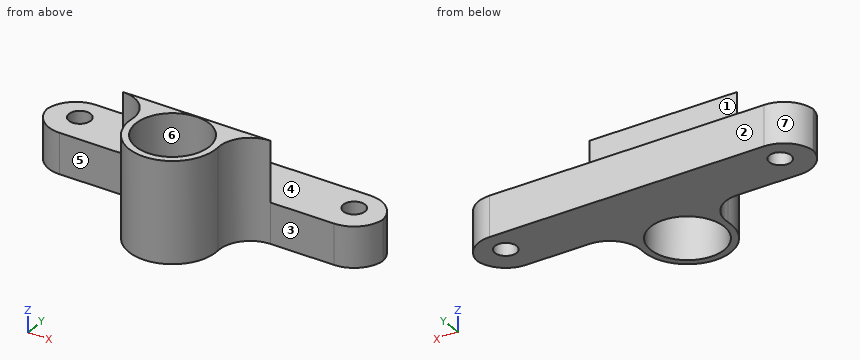
from build123d import *

# Parameters (mm, degrees)
F0_R     = 1.75
F0_R_2   = 5.9
F1_DEPTH = 6.5
F2_DEPTH = 16.2


with BuildPart() as f1:
    # F0 (on Top) → F1 (new body)
    with BuildSketch(Plane.XY):
        with BuildLine():
            Line((7.780111, 20.456612), (-36.719889, 20.456612))
            ThreePointArc((-36.719889, 20.456612), (-40.073991, 19.164712), (-41.694827, 15.956612))
            ThreePointArc((-41.694827, 15.956612), (-40.073991, 12.748513), (-36.719889, 11.456612))
            Line((-36.719889, 11.456612), (-26.42815, 11.456612))
            Line((-26.42815, 11.456612), (-2.511629, 11.456612))
            Line((-2.511629, 11.456612), (7.780111, 11.456612))
            ThreePointArc((7.780111, 11.456612), (11.134213, 12.748513), (12.755048, 15.956612))
            ThreePointArc((12.755048, 15.956612), (11.134213, 19.164712), (7.780111, 20.456612))
        make_face()
        with Locations((-36.719889, 16.456612)):
            Circle(F0_R, mode=Mode.SUBTRACT)
        with Locations((7.780111, 16.456612)):
            Circle(F0_R, mode=Mode.SUBTRACT)
        with BuildLine():
            Line((-2.511629, 11.456612), (-26.42815, 11.456612))
            ThreePointArc((-26.42815, 11.456612), (-22.74825, 9.841628), (-21.445541, 6.039946))
            ThreePointArc((-21.445541, 6.039946), (-14.469889, -1.543388), (-7.494237, 6.039946))
            ThreePointArc((-7.494237, 6.039946), (-6.191529, 9.841628), (-2.511629, 11.456612))
        make_face()
        with Locations((-14.469889, 5.456612)):
            Circle(F0_R_2, mode=Mode.SUBTRACT)
    extrude(amount=F1_DEPTH)

    # F0 (on Top) → F2 (join)
    with BuildSketch(Plane.XY):
        with BuildLine():
            Line((-2.511629, 11.456612), (-26.42815, 11.456612))
            ThreePointArc((-26.42815, 11.456612), (-22.74825, 9.841628), (-21.445541, 6.039946))
            ThreePointArc((-21.445541, 6.039946), (-14.469889, -1.543388), (-7.494237, 6.039946))
            ThreePointArc((-7.494237, 6.039946), (-6.191529, 9.841628), (-2.511629, 11.456612))
        make_face()
        with Locations((-14.469889, 5.456612)):
            Circle(F0_R_2, mode=Mode.SUBTRACT)
    extrude(amount=F2_DEPTH)


solid = f1.part
The listing builds one solid part. Answer for the finished solid, in the listing's coordinates (mm). Face numbers are marked on the shaded views. A direction names the side the tool comes from. Give positions to 0.01 mm unless a question says otherwise; leave off trailing zeros. Loops run counter-clockwise (first coordinate to the right, second up) from the corner with the lowest first, then second, coordinate; pieces in that order, holes last. Notation, with made-up numbers: (73, 38.25) - (90, 38.25) arc R17 cw to (90, 56.25) - close; hole circle Ø5 at (68.25, 0.5). An arc over 180 degrees is marked (long way). Answer as a JSON object with one key per item and string values.
1. A cutting plane is placed at D-D (y = 17). Write down the section's boundary in (x, z), then the cut area to 3 significant figures.
Determined:
{"outline": "(-41.48, 0) - (-38.38, 0) - (-38.38, 6.5) - (-41.48, 6.5) - close; (-35.06, 0) - (6.12, 0) - (6.12, 6.5) - (-35.06, 6.5) - close; (9.44, 0) - (12.54, 0) - (12.54, 6.5) - (9.44, 6.5) - close", "area": "308 mm²"}
2. For the marked faces 1, 2 and 3, determine the directions among +Z, -Z, +X, -X, +Y, -Y from which every point of the face is accessible in a straight line to the end or side of a thin tool.
Determined:
{"face 1": "+Z, +X, -X, +Y", "face 2": "+Z, -Z, +X, -X, +Y", "face 3": "+Z, -Z, +X, -Y"}
3. Find the intervals of material crossed by L1, parallel to Z at x = 2.5, y = 14.25; L2, parallel to X at y = 2.5, z = 14.5; L3, parallel to Y at x = -34.5, z = 4.75, in increasing order. Write a range as [from, to].
Determined:
{"L1": "[0, 6.5]", "L2": "[-20.81, -19.58], [-9.36, -8.12]", "L3": "[11.46, 20.46]"}
4. A cutting plane is placed at C-C (z = 7.5). Write down the section's boundary in (x, y).
Determined:
{"outline": "(-26.43, 11.46) arc R5 cw to (-21.45, 6.04) arc R7 ccw (long way) to (-7.49, 6.04) arc R5 cw to (-2.51, 11.46) - close; hole circle Ø11.8 at (-14.47, 5.46)"}
5. For a pull along Y with two mould halves and no side action, classify the marked faces 4, 5, 6 and 7 as pulls with the +Y half, pulls with the -Y half, needs draft (parallel to the pull), parting line crosses it, or undercut.
Determined:
{"face 4": "needs draft", "face 5": "pulls with the -Y half", "face 6": "undercut", "face 7": "pulls with the +Y half"}
6. A cutting plane is placed at A-A (y = 0.5). Write down the section's boundary in (x, z).
Determined:
{"outline": "(-19.41, 0) - (-17.67, 0) - (-17.67, 16.2) - (-19.41, 16.2) - close; (-11.27, 0) - (-9.53, 0) - (-9.53, 16.2) - (-11.27, 16.2) - close"}
7. Flat-ended cylindrical pins translate along their axes: pin 1 Ø2.5 at (x, y) = (-5, 14.5) entering from +Z; pin 2 Ø5.5 at (x, y) = (-36.72, 16.46) entering from -Z; pin 3 Ø1 at (y, z) = (1.5, 11) entering from -X; pin 4 Ø5 at (x, z) = (-13, 10.5) entering from +Y. Find the tip coordinate at first contact, or state that the pin passes through.
Determined:
{"pin 1": "z = 6.5", "pin 2": "z = 0", "pin 3": "x = -20.56", "pin 4": "y = 11.46"}
8. A cutting plane is placed at B-B (x = 9). Write down the section's boundary in (y, z), then the cut area to 3 significant figures.
Determined:
{"outline": "(11.61, 0) - (15.2, 0) - (15.2, 6.5) - (11.61, 6.5) - close; (17.71, 0) - (20.31, 0) - (20.31, 6.5) - (17.71, 6.5) - close", "area": "40.2 mm²"}
